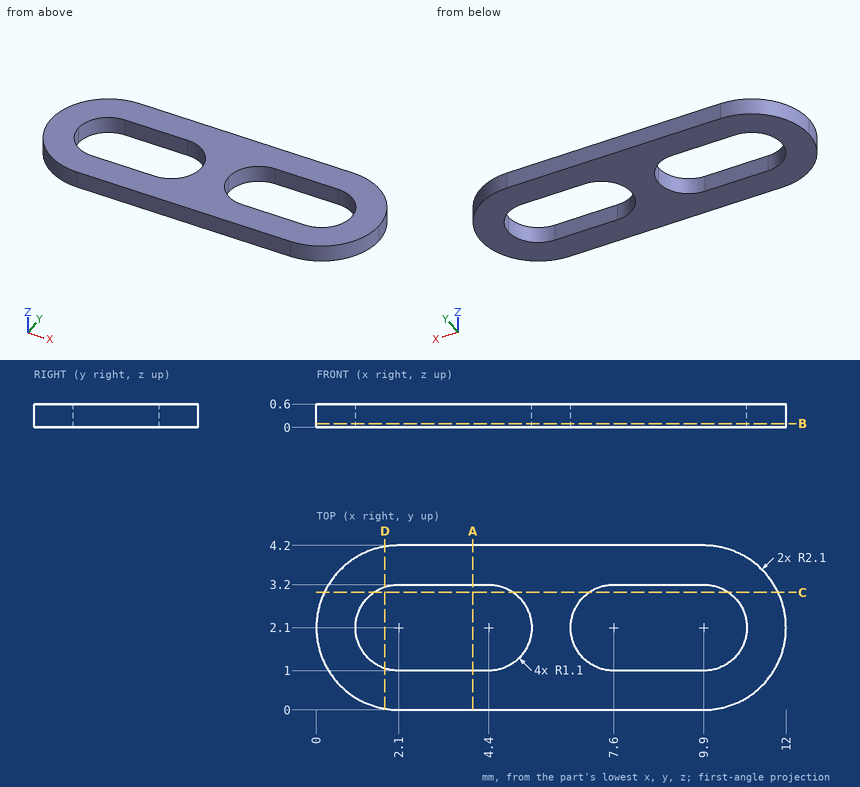
The drawing under review shows one solid part. Ordinate dimensions are in mm from its lowest x, y, z. Round coordinates to 2 decimals unless told otherwise and drop trailing zeros. Loops run counter-clockwise (first coordinate to the right, second up) from the corner with the lowest first, then second, coordinate; pieces in that order, holes last. Notation, with made-up numbers: (46.5, -10.5) - (99.5, -10.5) arc R30 ccw to (99.5, 16.5) - close; hole circle Ø8 at (-3, 20.5). An arc over 180 degrees is marked (long way). Use a Markdown table: item, result. Add a question column.
Q1. Add section A-A (x = 4). State the section outline as (y, z) points, plus the area to 3 significant figures.
Q2. Add section B-B (z = 0.1). State the section outline as (x, y) points.
Q3. Add section C-C (y = 3). State the section outline as (x, z) points, plus the area to 3 significant figures.
Q4. For probe 1 along Y at (x, z) = (9.5, 0.15); probe 2 along X at (y, z) = (2.6, 0.55); probe 3 along X at (y, z) = (1.1, 0.2), list the stretches that pass through material, from the lowest coordinate up.
Q5. Add section D-D (x = 1.75). State the section outline as (y, z) points.
Worked answers:
| question | item | result |
|---|---|---|
| 1 | outline | (0, 0) - (1, 0) - (1, 0.6) - (0, 0.6) - close; (3.2, 0) - (4.2, 0) - (4.2, 0.6) - (3.2, 0.6) - close |
| 1 | area | 1.20 mm² |
| 2 | outline | (0, 2.1) arc R2.1 ccw to (2.1, 0) - (9.9, 0) arc R2.1 ccw to (12, 2.1) arc R2.1 ccw to (9.9, 4.2) - (2.1, 4.2) arc R2.1 ccw to start; hole (1, 2.1) arc R1.1 ccw to (2.1, 1) - (4.4, 1) arc R1.1 ccw to (5.5, 2.1) arc R1.1 ccw to (4.4, 3.2) - (2.1, 3.2) arc R1.1 ccw to start; hole (6.5, 2.1) arc R1.1 ccw to (7.6, 1) - (9.9, 1) arc R1.1 ccw to (11, 2.1) arc R1.1 ccw to (9.9, 3.2) - (7.6, 3.2) arc R1.1 ccw to start |
| 3 | outline | (0.2, 0) - (1.47, 0) - (1.47, 0.6) - (0.2, 0.6) - close; (5.03, 0) - (6.97, 0) - (6.97, 0.6) - (5.03, 0.6) - close; (10.53, 0) - (11.8, 0) - (11.8, 0.6) - (10.53, 0.6) - close |
| 3 | area | 2.68 mm² |
| 4 | probe 1 | 0 to 1, 3.2 to 4.2 |
| 4 | probe 2 | 0.06 to 1.12, 5.38 to 6.62, 10.88 to 11.94 |
| 4 | probe 3 | 0.25 to 1.64, 4.86 to 7.14, 10.36 to 11.75 |
| 5 | outline | (0.03, 0) - (1.06, 0) - (1.06, 0.6) - (0.03, 0.6) - close; (3.14, 0) - (4.17, 0) - (4.17, 0.6) - (3.14, 0.6) - close |
